Could you check a few things on this model? Use its own coordinates, in mm. A direction names the side the tool comes from. Round coordinates to 2 decimals unless told otherwise and drop trailing zeros. Loops run counter-clockwise (first coordinate to the right, second up) from the corner with the lowest first, then second, coordinate; pieces in that order, holes last. Notation, with made-up numbers: (15, 88) - (43, 88) arc R12 ccw to (43, 96) - close; hole circle Ø10 at (-39.75, -36.5). An arc over 180 degrees is marked (long way). Put each result on its own line as item: value. Start each with the question number.
from build123d import *

# Parameters (mm, degrees)
SCHIZZO1_R                   = 22
SCHIZZO1_W                   = 51
SCHIZZO1_H                   = 102
SCHIZZO1_W_2                 = 31.947441117
SCHIZZO1_H_2                 = 22
ESTRUSIONE_ESTRUSIONE2_DEPTH = 82
SCHIZZO2_W                   = 80.086203662
SCHIZZO2_H                   = 68.356722048
TAGLIO_ESTRUSIONE1_DEPTH     = 6
SCHIZZO3_W                   = 81.899638904
SCHIZZO3_H                   = 77.244744974
TAGLIO_ESTRUSIONE4_DEPTH     = 16
ESTRUSIONE_ESTRUSIONE3_DEPTH = 22
SCHIZZO6_W                   = 102
SCHIZZO6_H                   = 22
ESTRUSIONE_ESTRUSIONE4_DEPTH = 44
SCHIZZO7_R                   = 8
TAGLIO_ESTRUSIONE5_DEPTH     = 130.452694062
SCHIZZO8_R                   = 12.5
TAGLIO_ESTRUSIONE6_DEPTH     = 139.29678232
SCHIZZO9_R                   = 12
TAGLIO_ESTRUSIONE7_DEPTH     = 130.452694062
RACCORDO1_R                  = 3
RACCORDO2_R                  = 3


with BuildPart() as part:
    # Schizzo1 → Estrusione-Estrusione2 (new body)
    with BuildSketch(Plane(origin=(0, 0, 0), x_dir=(1, 0, 0), z_dir=(0, 1, 0))):
        with Locations((77, 0)):
            Circle(SCHIZZO1_R)
        with Locations((0.5, 0)):
            Rectangle(SCHIZZO1_W, SCHIZZO1_H)
        with Locations((41.973720559, 0)):
            Rectangle(SCHIZZO1_W_2, SCHIZZO1_H_2)
    extrude(amount=ESTRUSIONE_ESTRUSIONE2_DEPTH)

    # Schizzo2 → Taglio-Estrusione1 (cut)
    with BuildSketch(Plane.XZ):
        with Locations((66.043101831, -4.044394055)):
            Rectangle(SCHIZZO2_W, SCHIZZO2_H)
    extrude(amount=-TAGLIO_ESTRUSIONE1_DEPTH, mode=Mode.SUBTRACT)

    # Schizzo3 → Taglio-Estrusione4 (cut)
    with BuildSketch(Plane(origin=(0, 82, 0), x_dir=(1, 0, 0), z_dir=(0, 1, 0))):
        with Locations((66.949819452, -1.56539862)):
            Rectangle(SCHIZZO3_W, SCHIZZO3_H)
    extrude(amount=-TAGLIO_ESTRUSIONE4_DEPTH, mode=Mode.SUBTRACT)

    # Schizzo5 → Estrusione-Estrusione3 (add)
    with BuildSketch(Plane.XY.offset(11)):
        Polygon((57.947441117, 66), (26, 82), (26, 66), align=None)
    extrude(amount=-ESTRUSIONE_ESTRUSIONE3_DEPTH)

    # Schizzo6 → Estrusione-Estrusione4 (add)
    with BuildSketch(Plane.ZY.offset(25)):
        with Locations((0, 55)):
            Rectangle(SCHIZZO6_W, SCHIZZO6_H)
    extrude(amount=ESTRUSIONE_ESTRUSIONE4_DEPTH)

    # Schizzo7 → Taglio-Estrusione5 (cut, through all)
    with BuildSketch(Plane(origin=(0, 66, 0), x_dir=(1, 0, 0), z_dir=(0, 1, 0))):
        with Locations(Location((-54, -25, 0), (0, 0, 270))):
            Circle(SCHIZZO7_R)
        with Locations(Location((-54, 25, 0), (0, 0, 270))):
            Circle(SCHIZZO7_R)
        Polygon((-25, -51), (-69, -44), (-69, -51), align=None)
        Polygon((-25, 51), (-69, 44), (-69, 51), align=None)
    extrude(amount=-TAGLIO_ESTRUSIONE5_DEPTH, mode=Mode.SUBTRACT)

    # Schizzo8 → Taglio-Estrusione6 (cut, through all)
    with BuildSketch(Plane(origin=(0, 82, 0), x_dir=(1, 0, 0), z_dir=(0, 1, 0))):
        with Locations(Location((0, -26, 0), (0, 0, 270))):
            Circle(SCHIZZO8_R)
        with Locations(Location((0, 26, 0), (0, 0, 270))):
            Circle(SCHIZZO8_R)
    extrude(amount=-TAGLIO_ESTRUSIONE6_DEPTH, mode=Mode.SUBTRACT)

    # Schizzo9 → Taglio-Estrusione7 (cut, through all)
    with BuildSketch(Plane(origin=(0, 66, 0), x_dir=(1, 0, 0), z_dir=(0, 1, 0))):
        with Locations(Location((77, 0, 0), (0, 0, 270))):
            Circle(SCHIZZO9_R)
    extrude(amount=-TAGLIO_ESTRUSIONE7_DEPTH, mode=Mode.SUBTRACT)

    # Raccordo1
    raccordo1_edges = [part.edges().sort_by_distance(p)[0] for p in [
        (26, 44, -11),
    ]]
    fillet(raccordo1_edges, radius=RACCORDO1_R)

    # Raccordo2
    # the kernel refuses this fillet: 3 mm, written as the material it adds along each edge
    with BuildSketch(Plane(origin=(26, 82, 11), x_dir=(1, 0, 0), z_dir=(0, -1, 0))) as raccordo2_piece_1_section:
        with BuildLine():
            CenterArc((RACCORDO2_R, RACCORDO2_R), RACCORDO2_R, 180, 90)
            Line((0, RACCORDO2_R), (0, 0))
            Line((0, 0), (RACCORDO2_R, 0))
        make_face()
    raccordo2_piece_1 = extrude(amount=76, mode=Mode.PRIVATE)
    raccordo2_piece_1 = split(raccordo2_piece_1, bisect_by=Plane(origin=(41.823834569, 74.075066289, 11.680808527), z_dir=(-0.44780189792218816, -0.8941327978646608, 0)), keep=Keep.TOP, mode=Mode.PRIVATE)
    add(raccordo2_piece_1)


solid = part.part
Item 1: Suppose I cut it at A-A, the plane y = 8. List the corners of the cut face in (x, z) for me, then the cut area to 3 significant figures.
Item 2: Thinking about a two-plate mould opening in X: for faces 5 (the face through (43, 44, -11)), 6 (the face through (-25, 74, 1)), 7 (the face through (0, 82, -1)), which applies, released by +X, released by -X, zero draft, split by the parting line, or undercut?
Item 3: I need wall thicknesses on line 1 (X direction, y = 25.5, z = 0); line 2 (Z direction, x = 4, y = 78.5); line 3 (Z direction, x = -56, y = 45.5). Which ranges of each line are inside material? Lowest first, please. Write a range as from..to.
Item 4: Will these pins go through, and if not, where does the flat tip stop? P1, Ø13, axis at x = -57, z = 4, coming from the +Y side; P2, Ø18.5, axis at x = -54, z = 25, coming from the -Y side; P3, Ø12, axis at y = 19, z = -19.5, coming from the +X side; P4, Ø12.5, axis at x = 80, z = -0.5, coming from the +Y side.
Item 5: Suppose I cut it at D-D, the plane z = -25. List the corners of the cut face in (x, y) for me.
Item 6: Suppose I cut it at B-B, the plane x = 0. List the corners of the cut face in (y, z) for me, then the cut area to 3 significant figures.
Item 7: Suppose I cut it at C-C, the plane z = 0. List the corners of the cut face in (x, y) for me.
Item 8: On a 3-axis mill with a long thin cutter (end or side, diameter ignored), from which of +Z, -Z, +X, -X, +Y, -Y can I reach the whole of each face in a straight line? I mean faces 1 (the face through (69.1, 66, 9.5)), 2 (the face through (-47, 66, -1)), 3 (the face through (63, 6, 0)), 4 (the face through (-25, 22, 1)). Say none if no direction works.
Numbers:
1. outline: (-25, -51) - (26, -51) - (26, -14) arc R3 cw to (29, -11) - (57.95, -11) arc R22 ccw (long way) to (57.95, 11) - (29, 11) arc R3 cw to (26, 14) - (26, 51) - (-25, 51) - close; hole circle Ø25 at (0, -26); hole circle Ø25 at (0, 26); hole circle Ø24 at (77, 0)
1. area: 5,950 mm^2
2. face 5: undercut
2. face 6: released by -X
2. face 7: zero draft
3. line 1: -25..65, 89..99
3. line 2: -51..-37.84, -14.16..14.16, 37.84..51
3. line 3: -46.07..-32.75, -17.25..17.25, 32.75..46.07
4. P1: y = 66
4. P2: y = 44
4. P3: x = 94.37
4. P4: through
5. outline: (-69, 44) - (-62, 44) - (-62, 66) - (-69, 66) - close; (-46, 44) - (-25, 44) - (-25, 0) - (-12.46, 0) - (-12.46, 82) - (-25, 82) - (-25, 66) - (-46, 66) - close; (12.46, 0) - (26, 0) - (26, 82) - (12.46, 82) - close
6. outline: (0, -51) - (82, -51) - (82, -38.5) - (0, -38.5) - close; (0, -13.5) - (82, -13.5) - (82, 13.5) - (0, 13.5) - close; (0, 38.5) - (82, 38.5) - (82, 51) - (0, 51) - close
6. area: 4,260 mm^2
7. outline: (-69, 44) - (-25, 44) - (-25, 0) - (26, 0) - (26, 6) - (65, 6) - (65, 66) - (57.95, 66) - (26, 82) - (-25, 82) - (-25, 66) - (-69, 66) - close; (89, 6) - (99, 6) - (99, 66) - (89, 66) - close
8. face 1: +Z, -Z, +X, +Y
8. face 2: +Z, -Z, -X, +Y
8. face 3: +Z, -Z, +X, -Y
8. face 4: +Z, -Z, -X, -Y
